Read the model definition and answer for the solid it produces. Units are mm, in the model's axes. A direction names the side the tool comes from. Coordinates: 2 decimals unless noted, no trailing zeros. Write each loop counter-clockwise with the first axis right and the second up, starting at its lowest first coordinate (ties: lowest second). Pieces come first, ordered by that corner, then holes.
from build123d import *

# Parameters (mm, degrees)
ESQUISSE1_W             = 40
ESQUISSE1_H             = 30
BOSS_EXTRU_1_DEPTH      = 8
ENL_V_START             = -8
ESQUISSE2_R             = 8
ENL_V_MAT_EXTRU_1_DEPTH = 7
ESQUISSE3_W             = 40
ESQUISSE3_H             = 22
BOSS_EXTRU_2_DEPTH      = 8
ESQUISSE4_R             = 1.55
ENL_V_MAT_EXTRU_2_DEPTH = 8
ESQUISSE5_W             = 40
ESQUISSE5_H             = 43
BOSS_EXTRU_3_DEPTH      = 8
ESQUISSE6_W             = 31
ESQUISSE6_H             = 20
ENL_V_MAT_EXTRU_3_DEPTH = 8
BOSS_EXTRU_4_DEPTH      = 8
ESQUISSE8_R             = 1.75
ENL_V_MAT_EXTRU_4_DEPTH = 84.624159189
ESQUISSE9_R             = 7
ENL_V_MAT_EXTRU_5_DEPTH = 84.534424042
ESQUISSE10_R            = 1.65
ENL_V_MAT_EXTRU_6_DEPTH = 10
ESQUISSE11_R            = 1.65
ENL_V_MAT_EXTRU_7_DEPTH = 84.624159189
CHANFREIN1_SIZE         = 19
CONG_1_R                = 3


with BuildPart() as part:
    # Esquisse1 → Boss.-Extru.1 (new body)
    with BuildSketch(Plane.XY):
        with Locations((20, 15)):
            Rectangle(ESQUISSE1_W, ESQUISSE1_H)
    extrude(amount=BOSS_EXTRU_1_DEPTH)

    # Esquisse2 → Enlèv. mat.-Extru.1 (cut)
    with BuildSketch(Plane.XY.offset(8).offset(ENL_V_START)):
        with Locations((20, 15)):
            Circle(ESQUISSE2_R)
    extrude(amount=ENL_V_MAT_EXTRU_1_DEPTH, mode=Mode.SUBTRACT)

    # Esquisse3 → Boss.-Extru.2 (add)
    with BuildSketch(Plane.XY.offset(8)):
        with Locations((20, -11)):
            Rectangle(ESQUISSE3_W, ESQUISSE3_H)
    extrude(amount=-BOSS_EXTRU_2_DEPTH)

    # Esquisse4 → Enlèv. mat.-Extru.2 (cut)
    with BuildSketch(Plane.XY.offset(8).offset(ENL_V_START)):
        with Locations((30, -19)):
            Circle(ESQUISSE4_R)
        with Locations(Location((30, 1, 0), (0, 0, 180))):
            Circle(ESQUISSE4_R)
        with Locations((10, 1)):
            Circle(ESQUISSE4_R)
        with Locations(Location((10, -19, 0), (0, 0, 180))):
            Circle(ESQUISSE4_R)
    extrude(amount=ENL_V_MAT_EXTRU_2_DEPTH, mode=Mode.SUBTRACT)

    # Esquisse5 → Boss.-Extru.3 (add)
    with BuildSketch(Plane.XY.offset(8)):
        with Locations((20, 51.5)):
            Rectangle(ESQUISSE5_W, ESQUISSE5_H)
    extrude(amount=-BOSS_EXTRU_3_DEPTH)

    # Esquisse6 → Enlèv. mat.-Extru.3 (cut)
    with BuildSketch(Plane.XY.offset(8).offset(ENL_V_START)):
        with Locations((15.5, 63)):
            Rectangle(ESQUISSE6_W, ESQUISSE6_H)
    extrude(amount=ENL_V_MAT_EXTRU_3_DEPTH, mode=Mode.SUBTRACT)

    # Esquisse7 → Boss.-Extru.4 (add)
    with BuildSketch(Plane.XY.offset(8)):
        Polygon((0, 53), (-10, 53), (-10, 73), (-19, 73), (-19, 45), (0, 45), align=None)
    extrude(amount=-BOSS_EXTRU_4_DEPTH)

    # Esquisse8 → Enlèv. mat.-Extru.4 (cut, through all)
    with BuildSketch(Plane.XY.offset(8)):
        with Locations((35.5, 58.5)):
            Circle(ESQUISSE8_R)
        with Locations(Location((35.5, 68.5, 0), (0, 0, 180))):
            Circle(ESQUISSE8_R)
        with Locations((-14.5, 68.5)):
            Circle(ESQUISSE8_R)
        with Locations(Location((-14.5, 58.5, 0), (0, 0, 180))):
            Circle(ESQUISSE8_R)
    extrude(amount=-ENL_V_MAT_EXTRU_4_DEPTH, mode=Mode.SUBTRACT)

    # Esquisse9 → Enlèv. mat.-Extru.5 (cut, through all)
    with BuildSketch(Plane(origin=(0, 0, 7), x_dir=(-1, 0, 0), z_dir=(0, 0, -1))):
        with Locations((-20, 15)):
            Circle(ESQUISSE9_R)
    extrude(amount=-ENL_V_MAT_EXTRU_5_DEPTH, mode=Mode.SUBTRACT)

    # Esquisse10 → Enlèv. mat.-Extru.6 (cut)
    with BuildSketch(Plane(origin=(0, -22, 0), x_dir=(-1, 0, 0), z_dir=(0, -1, 0))):
        with Locations(Location((-20, -4, 0), (0, 0, 90))):
            Circle(ESQUISSE10_R)
        with Locations(Location((-36, -4, 0), (0, 0, 90))):
            Circle(ESQUISSE10_R)
    extrude(amount=-ENL_V_MAT_EXTRU_6_DEPTH, mode=Mode.SUBTRACT)

    # Esquisse11 → Enlèv. mat.-Extru.7 (cut, through all)
    with BuildSketch(Plane(origin=(0, 0, 0), x_dir=(-1, 0, 0), z_dir=(0, 0, -1))):
        with Locations((-35, 21)):
            Circle(ESQUISSE11_R)
        with Locations(Location((-5, 21, 0), (0, 0, 180))):
            Circle(ESQUISSE11_R)
        with Locations((-5, 9)):
            Circle(ESQUISSE11_R)
        with Locations(Location((-35, 9, 0), (0, 0, 180))):
            Circle(ESQUISSE11_R)
    extrude(amount=-ENL_V_MAT_EXTRU_7_DEPTH, mode=Mode.SUBTRACT)

    # Chanfrein1
    chanfrein1_edges = [part.edges().sort_by_distance(p)[0] for p in [
        (0, 45, 4),
    ]]
    chamfer(chanfrein1_edges, length=CHANFREIN1_SIZE - 0.0001)  # a hair under: the kernel refuses the full size

    # Congé1
    cong_1_edges = [part.edges().sort_by_distance(p)[0] for p in [
        (31, 53, 4),
        (-10, 53, 4),
    ]]
    fillet(cong_1_edges, radius=CONG_1_R)


solid = part.part
Item 1: The part is cut by section D-D (y = -15). Give the vertices of the cut face in (x, z), and give its area (3 significant figures).
Item 2: The part is cut by section A-A (y = 68.5). Give the vertices of the cut face in (x, z), and give its area (3 significant figures).
Item 3: Find the intervals of material crossed by probe 1 along Y at (x, z) = (5, 4.75); probe 2 along X at (y, z) = (66, 6.25); probe 3 along Y at (x, z) = (20, 4.25), in increasing order.
Item 4: Determine the mould class of faces 1 (the cylindrical face through (30.1, 53.86, 4.06)), 2 (the flat face through (-19, 59, 4)), 3 (the flat face through (17, 26, 8)) for opening direction X: +X half, -X half, draft (parallel to the pull), parting line (faces both ways), or undercut.
Item 5: For faces 4 (the flat face through (24, 9, 7)), 5 (the flat face through (20, -22, 2)), 6 (the flat face through (36, -12, 4)), 7 (the cylindrical face through (30.83, -17.69, 3.94)), 8 (the cylindrical face through (-9.14, 53.9, 3.94)), determine the directions among +Z, -Z, +X, -X, +Y, -Y from which every point of the face is accessible in a straight line to the end or side of a thin tool.
Item 6: The part is cut by section B-B (z = 4). State how many separate pieces and enclosed holes the cut face has, and give its area (3 significant figures).
Item 7: The part is cut by section C-C (x = 30). Give the vertices of the cut face in (y, z).
Item 8: Given pin 1 (1.5 mm diameter, centred on x = 30, z = 6.5, fed in from +Y); pin 2 (2 mm diameter, centred on x = 20, z = 4, fed in from +Y); pin 3 (3 mm diameter, centred on x = 30, y = -19, fed in from +Z), each flat-ended and moving along its own axis, determine where each tip first touches the part or whether it passes through.
Answer:
1. outline: (0, 0) - (40, 0) - (40, 8) - (0, 8) - close; hole circle Ø3.3 at (20, 4); hole circle Ø3.3 at (36, 4)
1. area: 303 mm2
2. outline: (-19, 0) - (-16.25, 0) - (-16.25, 8) - (-19, 8) - close; (-12.75, 0) - (-10, 0) - (-10, 8) - (-12.75, 8) - close; (31, 0) - (33.75, 0) - (33.75, 8) - (31, 8) - close; (37.25, 0) - (40, 0) - (40, 8) - (37.25, 8) - close
2. area: 88.0 mm2
3. probe 1: y = -22 to 7.35, 10.65 to 19.35, 22.65 to 53
3. probe 2: x = -19 to -10, 31 to 40
3. probe 3: y = -12 to 7, 23 to 53
4. face 1: undercut
4. face 2: -X half
4. face 3: draft
5. face 4: -Z
5. face 5: +Z, -Z, +X, -X, -Y
5. face 6: -Y
5. face 7: +Z, -Z
5. face 8: +Z, -Z, +Y
6. separate pieces: 1
6. enclosed holes: 13
6. area: 3,330 mm2
7. outline: (-22, 0) - (-20.55, 0) - (-20.55, 8) - (-22, 8) - close; (-17.45, 0) - (-0.55, 0) - (-0.55, 8) - (-17.45, 8) - close; (2.55, 0) - (53.76, 0) - (53.76, 8) - (2.55, 8) - close
8. pin 1: stops at y = 54.8
8. pin 2: stops at y = 53
8. pin 3: passes through
